from build123d import *

# Parameters (mm, degrees)
SKETCH2_R           = 5
BOSS_EXTRUDE1_DEPTH = 10
CUT_EXTRUDE1_DEPTH  = 5
SKETCH4_R           = 3
CUT_EXTRUDE2_DEPTH  = 5


with BuildPart() as part:
    # Sketch2 → Boss-Extrude1 (new body)
    with BuildSketch(Plane.XY):
        Circle(SKETCH2_R)
    extrude(amount=BOSS_EXTRUDE1_DEPTH)

    # Sketch3 → Cut-Extrude1 (cut)
    with BuildSketch(Plane(origin=(0, 0, 0), x_dir=(-1, 0, 0), z_dir=(0, 0, -1))):
        with BuildLine():
            Line((1.908838778, 0.596937618), (0.830860529, -1.81925006))
            ThreePointArc((0.830860529, -1.81925006), (-1.826466205, 0.814874961), (1.908838778, 0.596937618))
        make_face()
    extrude(amount=-CUT_EXTRUDE1_DEPTH, mode=Mode.SUBTRACT)

    # Sketch4 → Cut-Extrude2 (cut)
    with BuildSketch(Plane.XY.offset(10)):
        Circle(SKETCH4_R)
    extrude(amount=-CUT_EXTRUDE2_DEPTH, mode=Mode.SUBTRACT)


solid = part.part
Here's how the part is built. I have some questions about the finished solid (model axes, mm). A direction names the side the tool comes from. Give positions to 0.01 mm unless a question says otherwise; leave off trailing zeros. Order: outer loops, then holes, each group sorted by start corner. A loop starts at its lowest first (then second) coordinate and runs counter-clockwise, first axis right, second up. Notation, with made-up numbers: M 87.5,-3.75 L 110.5,-3.75 A12 cw 110.5,3.25 Z; hole C -29,-4 d2. An arc over 180 degrees is marked long. Answer as a JSON object with one key per item and string values. Group by question number.
1) Please list where these lines run through material, in increasing order: L1, parallel to Y at x = 0, z = 5.75; L2, parallel to Y at x = 0, z = 1.3; L3, parallel to Z at x = 2, y = 1.25. Write a range as [from, to].
2) Suppose I cut it at B-B, the plane y = -1.5. Write out the boundary of the cut face in (x, z), plus the area to 3 significant figures.
3) On a 3-axis mill with a long thin cutter (end or side, diameter ignored), from which of +Z, -Z, +X, -X, +Y, -Y can I reach the whole of each face in a straight line? I mean faces 5 (the cylindrical face through (-3, 0, 8)), 6 (the cylindrical face through (1.853, 0.753, 2.465)). Say none if no direction works.
4) Suppose I cut it at D-D, the plane x = 4.25. Write out the boundary of the cut face in (y, z).
5) We'd pull the mould along X, two halves only. Please class faces 1 (the flat face through (-1.4, -1.3, 5)), 2 (the flat face through (-1.38, -0.59, 2.46)), 3 (the flat face through (-0.1, -3.3, 10)), 4 (the cylindrical face through (-1.08, -4.88, 4.93)): pulls with the +X half, pulls with the -X half, needs draft (parallel to the pull), parting line crosses it, or undercut.
6) Suppose I cut it at A-A, the plane x = 0. Write out the boundary of the cut face in (y, z).
7) Suppose I cut it at C-C, the plane z = 2. Write out the boundary of the cut face in (x, y), plus the area to 3 significant figures.
Results found:
{
 "1": {"L1": "[-5, -3], [3, 5]", "L2": "[-5, -2], [2, 5]", "L3": "[0, 5]"},
 "2": {"outline": "M -4.77,0 L -0.97,0 L -0.97,5 L -2.6,5 L -2.6,10 L -4.77,10 Z; M 1.32,0 L 4.77,0 L 4.77,10 L 2.6,10 L 2.6,5 L 1.32,5 Z", "area": "57.9 mm²"},
 "3": {"face 5": "+Z", "face 6": "+Z, -Z"},
 "4": {"outline": "M -2.63,0 L 2.63,0 L 2.63,10 L -2.63,10 Z"},
 "5": {"face 1": "undercut", "face 2": "undercut", "face 3": "needs draft", "face 4": "parting line crosses it"},
 "6": {"outline": "M -5,0 L -2,0 L -2,5 L -3,5 L -3,10 L -5,10 Z; M 2,0 L 5,0 L 5,10 L 3,10 L 3,5 L 2,5 Z"},
 "7": {"outline": "C 0,0 d10; hole M -1.91,0.6 L -0.83,-1.82 A2 ccw long Z", "area": "66.9 mm²"}
}
